```python
from build123d import *

# Parameters (mm, degrees)
CROQUIS1_R              = 5
SALIENTE_EXTRUIR1_DEPTH = 40
CROQUIS2_R              = 5.5
CROQUIS2_R_2            = 3.75
SALIENTE_EXTRUIR2_DEPTH = 15
CORTAR_EXTRUIR1_START   = -30
CROQUIS3_R              = 3.75
CORTAR_EXTRUIR1_DEPTH   = 30
CROQUIS4_R              = 5.5
CROQUIS4_R_2            = 2.5
SALIENTE_EXTRUIR3_DEPTH = 2


with BuildPart() as part:
    # Croquis1 → Saliente-Extruir1 (new body)
    with BuildSketch(Plane.XY):
        Circle(CROQUIS1_R)
    extrude(amount=-SALIENTE_EXTRUIR1_DEPTH)

    # Croquis2 → Saliente-Extruir2 (add, symmetric)
    with BuildSketch(Plane(origin=(0, 0, 0), x_dir=(1, 0, 0), z_dir=(0, 1, 0))):
        with Locations(Location((0, 42.202107472, 0), (0, 0, 270))):
            Circle(CROQUIS2_R)
        with Locations(Location((0, 42.202107472, 0), (0, 0, 270))):
            Circle(CROQUIS2_R_2, mode=Mode.SUBTRACT)
    extrude(amount=SALIENTE_EXTRUIR2_DEPTH, both=True)

    # Croquis3 → Cortar-Extruir1 (cut)
    with BuildSketch(Plane(origin=(0, 15, 0), x_dir=(1, 0, 0), z_dir=(0, 1, 0)).offset(CORTAR_EXTRUIR1_START)):
        with Locations(Location((0, 42.202107472, 0), (0, 0, 270))):
            Circle(CROQUIS3_R)
    extrude(amount=CORTAR_EXTRUIR1_DEPTH, mode=Mode.SUBTRACT)

    # Croquis4 → Saliente-Extruir3 (add)
    with BuildSketch(Plane(origin=(0, 15, 0), x_dir=(1, 0, 0), z_dir=(0, 1, 0))):
        with Locations(Location((0, 42.202107472, 0), (0, 0, 270))):
            Circle(CROQUIS4_R)
        with Locations(Location((0, 42.202107472, 0), (0, 0, 270))):
            Circle(CROQUIS4_R_2, mode=Mode.SUBTRACT)
    saliente_extruir3 = extrude(amount=-SALIENTE_EXTRUIR3_DEPTH)

    # Simetría1: Saliente-Extruir3 across plane
    add(saliente_extruir3.mirror(Plane.ZX))


solid = part.part
```
Could you check a few things on this model? Use its own coordinates, in mm. A direction names the side the tool comes from. Coordinates: 2 decimals unless noted, no trailing zeros. Write each loop counter-clockwise with the first axis right and the second up, starting at its lowest first coordinate (ties: lowest second). Pieces come first, ordered by that corner, then holes. Notation, with made-up numbers: M -7.5,-1.75 L -1.5,-1.75 A30 ccw -1.5,32.25 Z; hole C 61.5,22.5 d1. An arc over 180 degrees is marked long. Answer as CSV lines item,"result". Start each with the question number.
1) Please list where these lines run through material, in increasing order: line 1 (X direction, y = 10.5, z = -42); line 2 (X direction, y = -7, z = -44.5); line 3 (Z direction, x = 1.75, y = -13.5). Write a range as from..to.
2) I want a section at C-C, the plane z = -28.5. Please give me the cut outline in (x, y).
3) For P1, Ø3, axis at y = -1, z = -17.5, coming from the +X side; P2, Ø6, axis at y = -3.5, z = -5.5, coming from the -X side; P3, Ø3, axis at x = -2, z = -19.5, coming from the +Y side, each with a flat end and sliding along its axis, tell me the tip position at first contact or that it passes through.
4) We'd pull the mould along X, two halves only. Please class faces 3 (the flat face through (3, -15, -42)), 4 (the cylindrical face through (-5, 0, -20)), 5 (the cylindrical face through (0.1, -14, -44.7)): +X half, -X half, draft (parallel to the pull), parting line (faces both ways), or undercut.
5) I want a section at D-D, the plane y = 8.5. Please give me the cut outline in (x, z).
6) I want a section at A-A, the plane x = 0. Please give me the cut outline in (y, z), and give its area (3 significant figures).
7) I want a section at B-B, the plane y = 0. Please give me the cut outline in (x, z).
8) For faces 1 (the flat face through (0, 13, -45)), 2 (the flat face through (3, 15, -42)), which set-ups out of +Z, -Z, +X, -X, +Y, -Y let a thin tool reach every point of the face, with its end or its side?
Data:
1,line 1,"x = -5.5..-3.74, 3.74..5.5"
1,line 2,"x = -5..-2.96, 2.96..5"
1,line 3,"z = -47.42..-43.99, -40.42..-36.99"
2,outline,"C 0,0 d10"
3,P1,"stops at x = 5"
3,P2,"stops at x = -4.97"
3,P3,"stops at y = 4.97"
4,face 3,"draft"
4,face 4,"parting line"
4,face 5,"undercut"
5,outline,"C 0,-42.2 d11; hole C 0,-42.2 d7.5"
6,outline,"M -15,-47.7 L 15,-47.7 L 15,-44.7 L 13,-44.7 L 13,-45.95 L -13,-45.95 L -13,-44.7 L -15,-44.7 Z; M -15,-39.7 L -13,-39.7 L -13,-38.45 L 13,-38.45 L 13,-39.7 L 15,-39.7 L 15,-36.7 L 5,-36.7 L 5,0 L -5,0 L -5,-36.7 L -15,-36.7 Z"
6,area,"482 mm^2"
7,outline,"M -5,-39.91 A5.5 ccw long 5,-39.91 L 5,0 L -5,0 Z; hole C 0,-42.2 d7.5"
8,face 1,"none"
8,face 2,"+Z, -Z, +X, -X, +Y"
